from build123d import *

# Parameters (mm, degrees)
SKETCH1_W                       = 22.225
SKETCH1_H                       = 44.45
MAIN_BODY_EXTRUDE_DEPTH         = 19.05
SKETCH2_W                       = 10.16
SKETCH2_H                       = 10.16
UPPER_FOOT_CONNECTION_CUT_DEPTH = 15.24


with BuildPart() as part:
    # Sketch1 → Main body extrude (new body)
    with BuildSketch(Plane(origin=(0, 0, 0), x_dir=(1, 0, 0), z_dir=(0, 1, 0))):
        with BuildLine():
            Line((22.225, 44.45), (22.225, 0))
            ThreePointArc((22.225, 0), (0, 22.225), (22.225, 44.45))
        make_face()
        with Locations((33.3375, 22.225)):
            Rectangle(SKETCH1_W, SKETCH1_H)
    extrude(amount=MAIN_BODY_EXTRUDE_DEPTH)

    # Sketch2 → Upper foot connection cut (cut)
    with BuildSketch(Plane(origin=(44.45, 0, 0), x_dir=(0, 0, -1), z_dir=(1, 0, 0))):
        with Locations((22.225, 9.525)):
            Rectangle(SKETCH2_W, SKETCH2_H)
    extrude(amount=-UPPER_FOOT_CONNECTION_CUT_DEPTH, mode=Mode.SUBTRACT)


solid = part.part
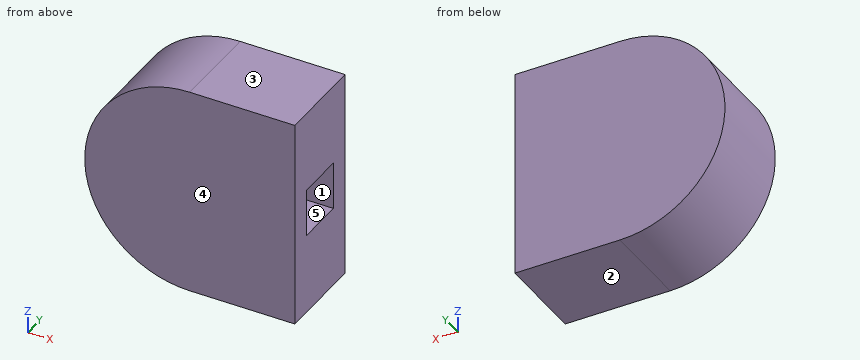
Read the model definition and answer for the solid it produces. Units are mm, in the model's axes. Face numbers are marked on the shaded views. A direction names the side the tool comes from. Round coordinates to 2 decimals unless told otherwise and drop trailing zeros. Order: outer loops, then holes, each group sorted by start corner. A loop starts at its lowest first (then second) coordinate and runs counter-clockwise, first axis right, second up.
1) The part is cut by section D-D on x = 13.5. Write down the section's boundary in (y, z), plus the area to 3 significant figures.
2) The part is cut by section C-C on z = -22.5. Write down the section's boundary in (x, y) (3 decimals), plus the area to 3 significant figures.
3) Straight lines are drawn through the part: L1, parallel to Z at x = 42, y = 7.75 (3 decimals); L2, parallel to Y at x = 35, z = -21 (3 decimals); L3, parallel to X at y = 1.25, z = -5. For each, find the intervals that lie inside material, in ascending order.
4) The part is cut by section A-A on x = 33. Write down the section's boundary in (y, z) (3 decimals), plus the area to 3 significant figures.
5) Flat-ended cylindrical pins translate along their axes: pin 1 (10 mm diameter, centred on x = 16.5, y = 11.5, fed in from +Z); pin 2 (4 mm diameter, centred on y = 8, z = -22, fed in from +X); pin 3 (8 mm diameter, centred on x = 33.5, z = -20, fed in from -Y); pin 4 (3 mm diameter, centred on y = 7, z = -29.5, fed in from -X). Find the tip coordinate at first contact, or state that the pin passes through.
6) The mould has two halves that part along Z. Classify the marked faces 1, 2 and 3: released by +Z, released by -Z, zero draft, split by the parting line, or undercut.
7) The part is cut by section B-B on y = 6.5. Write down the section's boundary in (x, z) (3 decimals).
8) For the marked faces 4 and 5, determine the directions among +Z, -Z, +X, -X, +Y, -Y from which every point of the face is accessible in a straight line to the end or side of a thin tool.
Resolved:
1. outline: (0, -42.67) - (19.05, -42.67) - (19.05, -1.78) - (0, -1.78) - close
1. area: 779 mm2
2. outline: (0.002, 0) - (44.45, 0) - (44.45, 4.445) - (29.21, 4.445) - (29.21, 14.605) - (44.45, 14.605) - (44.45, 19.05) - (0.002, 19.05) - close
2. area: 692 mm2
3. L1: z = -44.45 to -27.305, -17.145 to 0
3. L2: y = 0 to 4.445, 14.605 to 19.05
3. L3: x = 8.18 to 44.45
4. outline: (0, -44.45) - (19.05, -44.45) - (19.05, 0) - (0, 0) - close; hole (4.445, -27.305) - (14.605, -27.305) - (14.605, -17.145) - (4.445, -17.145) - close
4. area: 744 mm2
5. pin 1: stops at z = -0.01
5. pin 2: stops at x = 29.21
5. pin 3: stops at y = 0
5. pin 4: stops at x = 0.76
6. face 1: undercut
6. face 2: released by -Z
6. face 3: released by +Z
7. outline: (22.225, -44.45) - (44.45, -44.45) - (44.45, -27.305) - (29.21, -27.305) - (29.21, -17.145) - (44.45, -17.145) - (44.45, 0) - (22.225, 0) arc R22.225 ccw to start
8. face 4: +Z, -Z, +X, -X, -Y
8. face 5: +X
